```python
from build123d import *

# Parameters (mm, degrees)
SKETCH_1_W      = 3
SKETCH_1_H      = 10
SKETCH_1_H_2    = 12
EXTRUDE_1_DEPTH = 3
FILLET_1_R      = 3


with BuildPart() as part:
    # Эскиз1 → Бобышка-Вытянуть1 (new body)
    with BuildSketch(Plane(origin=(0, 0, 0), x_dir=(0, 0, -1), z_dir=(1, 0, 0))):
        Polygon((-26, 4), (13, 12), (26, 12), (26, -12), (-26, -12), align=None)
        with Locations((-21.5, -4)):
            Rectangle(SKETCH_1_W, SKETCH_1_H, mode=Mode.SUBTRACT)
        with Locations((21.5, 3)):
            Rectangle(SKETCH_1_W, SKETCH_1_H_2, mode=Mode.SUBTRACT)
    extrude(amount=EXTRUDE_1_DEPTH)

    # Скругление1
    fillet_1_edges = [part.edges().sort_by_distance(p)[0] for p in [
        (1.5, 4, 26),
        (1.5, 12, -13),
        (1.5, 12, -26),
        (1.5, -12, -26),
        (1.5, -12, 26),
    ]]
    fillet(fillet_1_edges, radius=FILLET_1_R)


solid = part.part
```
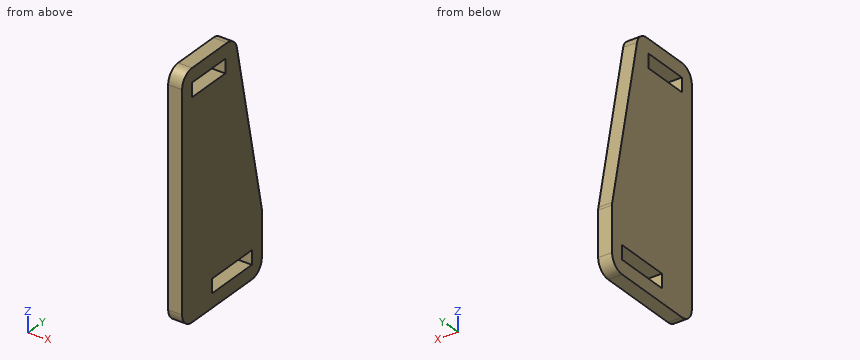
Can you work these out from the model? Positions are in its coordinate system, mm. Coordinates: 2 decimals unless noted, no trailing zeros. Loops run counter-clockwise (first coordinate to the right, second up) from the corner with the lowest first, then second, coordinate; pieces in that order, holes last.
1) Imagine slicing it at A-A on x = 0.9. List the corners of the cut face in (y, z) for me, plus the area to 3 significant figures.
2) Imagine slicing it at D-D on z = 6.5. List the corners of the cut face in (x, y) for me.
3) I need wall thicknesses on probe 1 along Z at (x, y) = (2.6, 0); probe 2 along Z at (x, y) = (0.85, -7.5); probe 3 along Y at (x, z) = (2, -12). Which ranges of each line are inside material? Lowest first, please.
4) For pin 1 (1.5 mm diameter, centred on x = 2, y = 2, fed in from +Z); pin 2 (0.9 mm diameter, centred on x = 1.5, z = 21.5, fed in from +Y); pin 3 (1 mm diameter, centred on x = 2, z = 1, fed in from +Y), each with a flat end and sliding along its axis, tell me the tip position at first contact or that it passes through.
5) Imagine slicing it at B-B on y = -6.5. List the corners of the cut face in (x, z) for me.
6) Imagine slicing it at C-C on y = 3.5. List the corners of the cut face in (x, z) for me, plus the area to 3 significant figures.
Completed:
1. outline: (-12, -23) arc R3 ccw to (-9, -26) - (9, -26) arc R3 ccw to (12, -23) - (12, -13.3) arc R3 ccw to (11.94, -12.7) - (4.49, 23.6) arc R3 ccw to (1.55, 26) - (-9, 26) arc R3 ccw to (-12, 23) - close; hole (-9, 20) - (1, 20) - (1, 23) - (-9, 23) - close; hole (-3, -23) - (9, -23) - (9, -20) - (-3, -20) - close
1. area: 1,020 mm2
2. outline: (0, -12) - (3, -12) - (3, 8) - (0, 8) - close
3. probe 1: z = -26 to -23, -20 to 20, 23 to 26
3. probe 2: z = -26 to 20, 23 to 26
3. probe 3: y = -12 to 11.79
4. pin 1: stops at z = 26
4. pin 2: stops at y = 5.02
4. pin 3: stops at y = 9.23
5. outline: (0, -26) - (3, -26) - (3, 20) - (0, 20) - close; (0, 23) - (3, 23) - (3, 26) - (0, 26) - close
6. outline: (0, -26) - (3, -26) - (3, -23) - (0, -23) - close; (0, -20) - (3, -20) - (3, 25.28) - (0, 25.28) - close
6. area: 145 mm2
